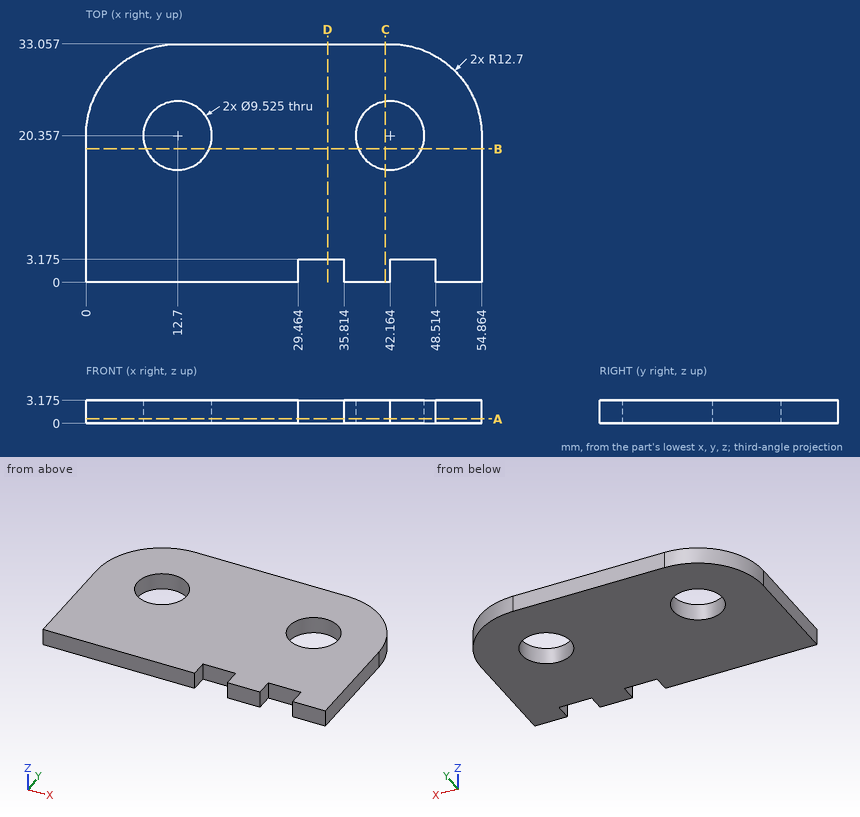
Can you work these out from the drawing? Everything is in mm from the part's minimum corner. Round coordinates to 2 decimals unless told otherwise and drop trailing zeros. Write each loop counter-clockwise with the first axis right and the second up, starting at its lowest first coordinate (ties: lowest second). Pieces come first, ordered by that corner, then holes. Notation, with made-up numbers: (3.25, 41.5) - (41.25, 41.5) arc R20 ccw to (41.25, 50.5) - close; hole circle Ø5 at (-35, 43). An arc over 180 degrees is marked (long way). Put each result on its own line as item: value. Start each with the question number.
(1) I want a section at C-C, the plane x = 41.5. Please give me the cut outline in (y, z) (1 decimal).
(2) Will this pin go through, and if not, where does the flat tip stop? pin 1 (12 mm diameter, centred on x = 22.5, y = 7, fed in from -Z).
(3) I want a section at D-D, the plane x = 33.5. Please give me the cut outline in (y, z) (1 decimal).
(4) I want a section at B-B, the plane y = 18.5. Please give me the cut outline in (x, z) (1 decimal).
(5) I need wall thicknesses on probe 1 along Y at (x, z) = (12.7, 1.4); probe 2 along X at (y, z) = (22, 2.4); probe 3 along X at (y, z) = (22.5, 1.9). Which ranges of each line are inside material? Lowest first, please.
(6) I want a section at A-A, the plane z = 0.6. Please give me the cut outline in (x, y) (1 decimal).
Here are the results:
1. outline: (0, 0) - (15.6, 0) - (15.6, 3.2) - (0, 3.2) - close; (25.1, 0) - (33.1, 0) - (33.1, 3.2) - (25.1, 3.2) - close
2. pin 1: stops at z = 0
3. outline: (3.2, 0) - (33.1, 0) - (33.1, 3.2) - (3.2, 3.2) - close
4. outline: (0, 0) - (8.3, 0) - (8.3, 3.2) - (0, 3.2) - close; (17.1, 0) - (37.8, 0) - (37.8, 3.2) - (17.1, 3.2) - close; (46.5, 0) - (54.9, 0) - (54.9, 3.2) - (46.5, 3.2) - close
5. probe 1: y = 0 to 15.59, 25.12 to 33.06
5. probe 2: x = 0.11 to 8.23, 17.17 to 37.69, 46.63 to 54.76
5. probe 3: x = 0.18 to 8.45, 16.95 to 37.91, 46.42 to 54.68
6. outline: (0, 0) - (29.5, 0) - (29.5, 3.2) - (35.8, 3.2) - (35.8, 0) - (42.2, 0) - (42.2, 3.2) - (48.5, 3.2) - (48.5, 0) - (54.9, 0) - (54.9, 20.4) arc R12.7 ccw to (42.2, 33.1) - (12.7, 33.1) arc R12.7 ccw to (0, 20.4) - close; hole circle Ø9.5 at (12.7, 20.4); hole circle Ø9.5 at (42.2, 20.4)
